The model under review builds one solid part; all positions refer to its coordinate system, in mm. A direction names the side the tool comes from. Round coordinates to 2 decimals unless told otherwise and drop trailing zeros. Order: outer loops, then holes, each group sorted by start corner. A loop starts at its lowest first (then second) coordinate and runs counter-clockwise, first axis right, second up.
1) Consider section C-C (x = 16). Give the boundary of the cut face in (y, z).
2) Mouldability with a two-part tool opening along Y and no side actions: class faces 5 (the face through (324.65, -66.21, 394.68)), 6 (the face through (324.65, -593.51, 107.09)), 7 (the face through (324.65, 53.911, 87.175)), 8 (the face through (-4.2, 284.729, 877.965)) as pulls with the +Y half, pulls with the -Y half, needs draft (parallel to the pull), parting line crosses it, or undercut.
3) Clearance check with flat-ended pins moving along their axes: P1, Ø1, axis at x = 162, z = 482, coming from the +Y side; P2, Ø5, axis at x = -245, z = 220, coming from the +Y side; P3, Ø8, axis at x = 140, z = 486, coming from the -Y side. State where each tip first meets the part, or that it passes through.
4) Consider section B-B (z = 281.5). Give the boundary of the cut face in (x, y).
5) Machinability: for faces 1 (the face through (-300, -647, -107)), 2 (the face through (300, -647, 124)), 3 (the face through (-300, 201, 462)), 4 (the face through (-325.35, 53.911, 87.175)), which of the approach directions +Z, -Z, +X, -X, +Y, -Y give a long, thin tool a straight path to every point of the face, cutting with its end or side? Answer none if there is none.
6) Consider section D-D (z = -84). Give the boundary of the cut face in (x, y).
7) To check wall thickness, follow L1, parallel to Z at x = -60.5, y = -96; L2, parallel to Z at x = 101, y = -136; L3, parallel to X at y = 247, z = 433. State the ranges of each line that lie inside material, in increasing order.
8) Consider section A-A (y = -209.5). Give the boundary of the cut face in (x, z).
Autodesk Fusion 360 part; units mm, degrees
sketch "草图1" plane through (0, 0, 0) normal (1, 0, 0) x (0, 1, 0)
  line L0 (-649.2476, 0) -> (0, 0)
  arc A0 (0, 0) -> (270.8221, 227.2465) centre (0, 275) ccw
  line L1 (270.8221, 227.2465) -> (373.8385, 811.4816)
  arc A1 (373.8385, 811.4816) -> (333.2805, 869.4044) centre (324.5981, 820.164) ccw
  line L2 (333.2805, 869.4044) -> (234.7997, 886.7692)
  arc A2 (234.7997, 886.7692) -> (176.8769, 846.2112) centre (226.1173, 837.5288) ccw
  line L3 (176.8769, 846.2112) -> (92.3655, 366.9231)
  arc A3 (-106.5657, 200) -> (92.3655, 366.9231) centre (-106.5657, 402) ccw
  line L4 (-106.5657, 200) -> (-649.2476, 200)
  arc A4 (-649.2476, 200) -> (-699.2476, 150) centre (-649.2476, 150) ccw
  line L5 (-699.2476, 150) -> (-699.2476, 50)
  arc A5 (-699.2476, 50) -> (-649.2476, 0) centre (-649.2476, 50) ccw
  line L6 (-130, 0) -> (100, 0) construction
  line L7 (373.8385, 811.4816) -> (230.7524, 0) construction
  dimension "d1" = 200
  dimension "d2" = 50
  dimension "d3" = 50
  dimension "d4" = 100
  dimension "d5" = 930
  dimension "d6" = 874
  dimension "d7" = 50
  dimension "d8" = 50
  dimension "d9" = 275
  dimension "d10" = 202
  dimension "d11" = 200
extrude "拉伸1" add sketch "草图1" along normal mid plane 600 makes body 1
sketch "草图2" plane through (300, 0, 0) normal (1, 0, 0) x (0, 1, 0)
  line L0 (-1000, 0) -> (500, 0) construction
  line L1 (-255.2476, 500) -> (-255.2476, -500) construction
  line L2 (-699.2476, 150) -> (-699.2476, 50)
  line L3 (-699.2476, -200) -> (-663.2885, -200)
  line L4 (-663.2885, -200) -> (-468.2546, 366.4195)
  line L5 (-699.2476, -200) -> (-484.7688, 422.8917)
  arc A0 (-443.2224, 444.4975) -> (-484.7688, 422.8917) centre (-452.6211, 411.8224) ccw
  arc A1 (-408.5365, 399.5028) -> (-468.2546, 366.4195) centre (-420.0332, 349.8155) ccw
  arc A2 (-408.5365, 399.5028) -> (-101.9587, 399.5028) centre (-255.2476, 1062) ccw
  arc A3 (-443.2224, 444.4975) -> (-67.2728, 444.4975) centre (-255.2476, 1098) ccw
  arc A4 (-25.7264, 422.8917) -> (-67.2728, 444.4975) centre (-57.8741, 411.8224) ccw
  arc A5 (-42.2406, 366.4195) -> (-101.9587, 399.5028) centre (-90.462, 349.8155) ccw
  line L6 (-42.2406, 366.4195) -> (152.7933, -200)
  line L7 (152.7933, -200) -> (188.7524, -200)
  line L8 (188.7524, -200) -> (-25.7264, 422.8917)
  line L9 (-255.2476, 500) -> (-255.2476, 524.2021) construction
  line L10 (-255.2476, 524.2021) -> (-255.2476, 850) construction
  dimension "d16" = 444
  dimension "d17" = 34
  dimension "d18" = 888
  dimension "d19" = 34
  dimension "d20" = 34
  dimension "d21" = 680
  dimension "d22" = 51
  dimension "d23" = 51
  dimension "d24" = 36
  dimension "d25" = 38
  dimension "d26" = 200
  dimension "d27" = 418
  dimension "d28" = 680
extrude "拉伸2" add sketch "草图2" along normal blind 50 separate body makes body 2
copy_body "复制和粘贴实体1" bodies 2 makes body 3
move_body "移动1" bodies 3 to x (1, 0, 0) y (0, 1, 0) z (0, 0, 1) at (-650, 0, 0)
combine "合并1" operation add target body 1 tool bodies 3 2
Answer below:
1. outline: (-699.25, 50) arc R50 ccw to (-649.25, 0) - (0, 0) arc R275 ccw to (270.82, 227.25) - (373.84, 811.48) arc R50 ccw to (333.28, 869.4) - (234.8, 886.77) arc R50 ccw to (176.88, 846.21) - (92.37, 366.92) arc R202 cw to (-106.57, 200) - (-649.25, 200) arc R50 ccw to (-699.25, 150) - close
2. face 5: undercut
2. face 6: pulls with the -Y half
2. face 7: undercut
2. face 8: pulls with the +Y half
3. P1: stops at y = 315.83
3. P2: stops at y = 269.94
3. P3: stops at y = 112.66
4. outline: (-350, -533.45) - (-300, -533.45) - (-300, -497.49) - (-350, -497.49) - close; (-350, -13) - (-300, -13) - (-300, 22.96) - (-350, 22.96) - close; (-300, 55.56) - (300, 55.56) - (300, 280.39) - (-300, 280.39) - close; (300, -533.45) - (350, -533.45) - (350, -497.49) - (300, -497.49) - close; (300, -13) - (350, -13) - (350, 22.96) - (300, 22.96) - close
5. face 1: -Z, +Y, -Y
5. face 2: +Z, +X, -Y
5. face 3: +Z, -X, +Y
5. face 4: -Z, -X
6. outline: (-350, -659.31) - (-300, -659.31) - (-300, -623.35) - (-350, -623.35) - close; (-350, 112.85) - (-300, 112.85) - (-300, 148.81) - (-350, 148.81) - close; (300, -659.31) - (350, -659.31) - (350, -623.35) - (300, -623.35) - close; (300, 112.85) - (350, 112.85) - (350, 148.81) - (300, 148.81) - close
7. L1: z = 0 to 200.28
7. L2: z = 0 to 200
7. L3: x = -300 to 300
8. outline: (-350, 383.54) - (-300, 383.54) - (-300, 419.54) - (-350, 419.54) - close; (-300, 0) - (300, 0) - (300, 200) - (-300, 200) - close; (300, 383.54) - (350, 383.54) - (350, 419.54) - (300, 419.54) - close
